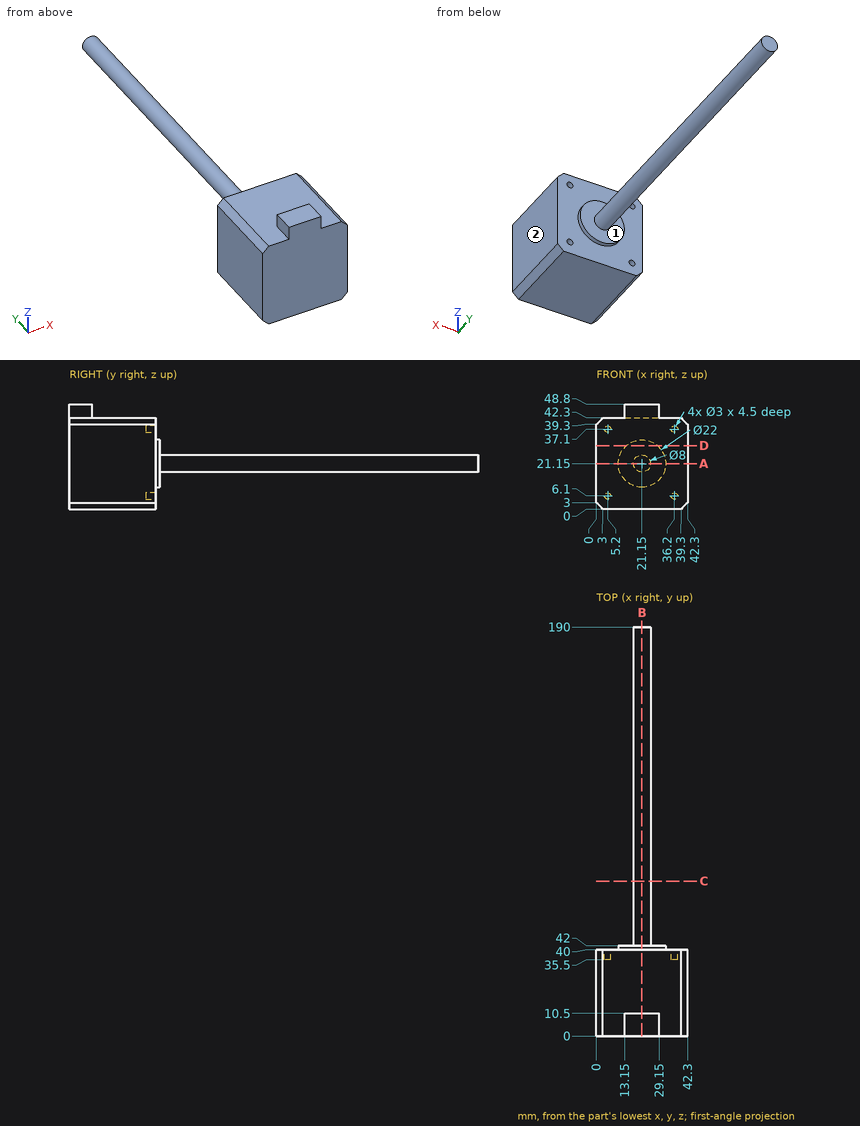
Verification items for this drawing (mm, ordinates from the low corner). A direction names the side the tool comes from. Give positions to 0.01 mm unless a question says otherwise; leave off trailing zeros. Write each loop counter-clockwise with the first axis right and the second up, starting at its lowest first coordinate (ties: lowest second). Pieces come first, ordered by that corner, then holes.
1) Access from +Z, -Z, +X, -X, +Y, -Y to the whole of each face (thin tool, end or side, straight path). Record for the marked faces 1 and 2.
2) Material ranges on L1, parallel to X at y = 39, z = 37; L2, parallel to Z at x = 5, y = 37; L3, parallel to Y at x = 34, z = 19, recorded low to high.
3) Section check C-C, the plane y = 72. Record the boundary of the cut face in (x, z), and give its area (3 significant figures).
4) Section check B-B, the plane x = 21.15. Record the boundary of the cut face in (y, z), and give its area (3 significant figures).
5) Gauge pin test, flat ends, axial feed: pin 1 (2.5 mm diameter, centred on x = 5.2, z = 6.1, fed in from +Y); pin 2 (3.5 mm diameter, centred on x = 35.5, z = 5.5, fed in from +Y); pin 3 (12.5 mm diameter, centred on x = 23.5, z = 17, fed in from +Y); pin 4 (11 mm diameter, centred on x = 17.5, y = 17, fed in from +Z). Record the tip position at first contact, or that the pin passes through.
6) Section check D-D, the plane z = 29.5. Record the boundary of the cut face in (x, y).
7) Section check A-A, the plane z = 21.15. Record the boundary of the cut face in (x, y), and give its area (3 significant figures).
Computed:
1. face 1: +Y
1. face 2: +Z, -Z, +X, +Y, -Y
2. L1: x = 0 to 3.7, 6.7 to 34.7, 37.7 to 42.3
2. L2: z = 0 to 4.61, 7.59 to 35.61, 38.59 to 42.3
2. L3: y = 0 to 40
3. outline: circle Ø8 at (21.15, 21.15)
3. area: 50.3 mm2
4. outline: (0, 0) - (40, 0) - (40, 10.15) - (42, 10.15) - (42, 17.15) - (190, 17.15) - (190, 25.15) - (42, 25.15) - (42, 32.15) - (40, 32.15) - (40, 42.3) - (10.5, 42.3) - (10.5, 48.8) - (0, 48.8) - close
4. area: 2,990 mm2
5. pin 1: stops at y = 35.5
5. pin 2: stops at y = 40
5. pin 3: stops at y = 190
5. pin 4: stops at z = 42.3
6. outline: (0, 0) - (42.3, 0) - (42.3, 40) - (28.31, 40) - (28.31, 42) - (13.99, 42) - (13.99, 40) - (0, 40) - close
7. outline: (0, 0) - (42.3, 0) - (42.3, 40) - (32.15, 40) - (32.15, 42) - (25.15, 42) - (25.15, 190) - (17.15, 190) - (17.15, 42) - (10.15, 42) - (10.15, 40) - (0, 40) - close
7. area: 2,920 mm2
